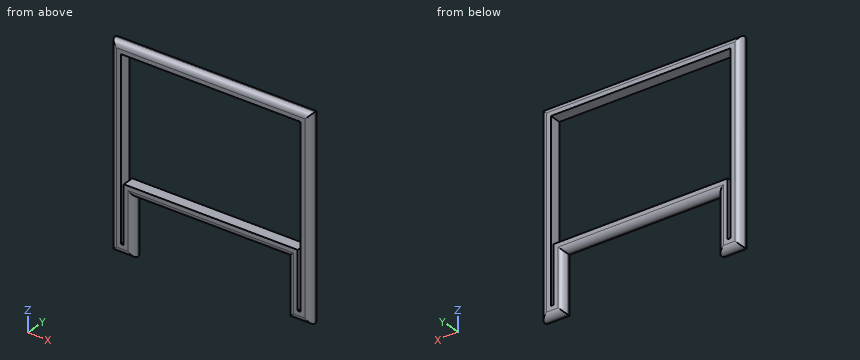
from build123d import *

# Parameters (mm, degrees)
BOSS_EXTRUDE1_DEPTH = 25.4
FILLET1_R           = 12.7


with BuildPart() as part:
    # Sketch2 → Boss-Extrude1 (new body)
    with BuildSketch(Plane(origin=(0, 0, 0), x_dir=(1, 0, 0), z_dir=(0, 1, 0))):
        Polygon((-219.925, -154.925), (219.925, -154.925), (219.925, 132.7), (219.925, 279.925000096), (169.125, 279.925000096), (169.125, 154.925), (-169.125, 154.925), (-169.125, 279.925000096), (-219.925, 279.925000096), (-219.925, 132.7), align=None)
        Polygon((-191.35, 132.7), (-191.35, 257.700000096), (-197.7, 257.700000096), (-197.7, 132.7), (-197.7, -132.7), (197.7, -132.7), (197.7, 132.7), (197.7, 257.700000096), (191.35, 257.700000096), (191.35, 132.7), align=None, mode=Mode.SUBTRACT)
    extrude(amount=BOSS_EXTRUDE1_DEPTH)

    # Fillet1
    fillet1_edges = [part.edges().sort_by_distance(p)[0] for p in [
        (0, 0, 154.925),
        (0, 25.4, 154.925),
        (-219.925, 0, -62.500000048),
        (-194.525, 0, -279.925000096),
        (-219.925, 25.4, -62.500000048),
        (-194.525, 25.4, -279.925000096),
        (-169.125, 0, -217.425000048),
        (-169.125, 25.4, -217.425000048),
        (0, 0, -154.925),
        (0, 25.4, -154.925),
        (219.925, 0, -62.500000048),
        (219.925, 25.4, -62.500000048),
        (194.525, 0, -279.925000096),
        (194.525, 25.4, -279.925000096),
        (169.125, 0, -217.425000048),
        (169.125, 25.4, -217.425000048),
    ]]
    fillet(fillet1_edges, radius=FILLET1_R - 0.0001)  # a hair under: the kernel refuses the full size


solid = part.part
Verification items for the finished model (mm, model axes). Coordinates: 2 decimals unless noted, no trailing zeros. Order: outer loops, then holes, each group sorted by start corner. A loop starts at its lowest first (then second) coordinate and runs counter-clockwise, first axis right, second up. Notation, with made-up numbers: (66.25, 22) -> (87.25, 22) arc R19 ccw to (87.25, 42) -> close; hole circle Ø1 at (-7.75, -13). An arc over 180 degrees is marked (long way). Put each result on its own line as item: value. Start each with the question number.
1. Go/stop test with flat-tipped pins: pin 1 Ø12.5 at (y, z) = (10, -72) entering from +X (3 decimals); pin 2 Ø1.9 at (x, y) = (195.5, 17.5) entering from +Z; pin 3 Ø3 at (y, z) = (17, 57) entering from +X; pin 4 Ø3 at (y, z) = (8.5, -104) entering from -X. Record where each tip stops, or that it passes through.
2. Cross-section at C-C, the plane y = 21.5. Record the boundary of the cut face in (x, z).
3. Material ranges on L1, parallel to X at y = 12, z = 32; L2, parallel to Z at x = -10, y = 13.5; L3, parallel to X at y = 8, z = -181, recorded low to high. Write a range as [from, to].
Computed:
1. pin 1: x = 219.925
1. pin 2: z = 154.33
1. pin 3: x = 219.61
1. pin 4: x = -219.63
2. outline: (-216.38, -276.38) -> (-172.67, -276.38) -> (-172.67, -151.38) -> (172.67, -151.38) -> (172.67, -276.38) -> (216.38, -276.38) -> (216.38, 151.38) -> (-216.38, 151.38) -> close; hole (-197.7, -257.7) -> (-191.35, -257.7) -> (-191.35, -132.7) -> (191.35, -132.7) -> (191.35, -257.7) -> (197.7, -257.7) -> (197.7, 132.7) -> (-197.7, 132.7) -> close
3. L1: [-219.91, -197.7], [197.7, 219.91]
3. L2: [-154.9, -132.7], [132.7, 154.9]
3. L3: [-219.02, -197.7], [-191.35, -170.03], [170.03, 191.35], [197.7, 219.02]
